Verification items for the finished model (mm, model axes). A direction names the side the tool comes from. Round coordinates to 2 decimals unless told otherwise and drop trailing zeros. Loops run counter-clockwise (first coordinate to the right, second up) from the corner with the lowest first, then second, coordinate; pieces in that order, holes last.
from build123d import *

# Parameters (mm, degrees)
F0_W     = 127
F0_H     = 127
F0_W_2   = 12.7
F0_H_2   = 101.6
F1_DEPTH = 12.7
F2_T     = -2.54


with BuildPart() as f1:
    # F0 (on Top) → F1 (new body)
    with BuildSketch(Plane.XY):
        with Locations((-24.9704163089, 19.614642486)):
            Rectangle(F0_W, F0_H)
        with Locations((-69.4204163089, 19.614642486)):
            Rectangle(F0_W_2, F0_H_2, mode=Mode.SUBTRACT)
        Polygon((-50.3704163089, 6.914642486), (-50.3704163089, 19.614642486), (-50.0745723798, 32.314642486), (-37.0573314681, 32.314642486), (-37.0573314681, 6.914642486), align=None, mode=Mode.SUBTRACT)
        Polygon((-31.3204163089, 32.314642486), (-24.9704163089, 32.314642486), (-18.6204163089, 32.314642486), (-18.6204163089, 6.914642486), (-31.3204163089, 6.914642486), align=None, mode=Mode.SUBTRACT)
        Polygon((0.4295836911, 32.314642486), (0.4295836911, 19.614642486), (0.4295836911, 6.914642486), (-10.8125778138, 6.914642486), (-10.8125778138, 32.314642486), align=None, mode=Mode.SUBTRACT)
        with Locations((19.4795836911, 19.614642486)):
            Rectangle(F0_W_2, F0_H_2, mode=Mode.SUBTRACT)
    extrude(amount=F1_DEPTH)

    # F2
    f2_openings = [f1.faces().sort_by_distance(p)[0] for p in [
        (36.733532, 19.614642, 12.7),
    ]]
    offset(amount=F2_T, openings=f2_openings, kind=Kind.INTERSECTION)


solid = f1.part
1. Scan lines: L1, parallel to X at y = 65.5, z = 10.5; L2, parallel to Y at x = 13.5, z = 5.5; L3, parallel to X at y = 11.5, z = 1.75. Record each from-to range of solid material in increasing order.
2. Section check A-A (y = -2). Enter the section's corners in (x, z).
3. Section check C-C (z = 8.5). Give the number of separate pieces and of enclosed holes in the cut face, then the cut area to 3 significant figures.
4. Release check for a two-part mould opening along X. For faces 4 (the face through (38.53, 19, 6)), 5 (the face through (-12, 21, 0)), 6 (the face through (-60.53, 19, 8)), 7 (the face through (-5, 32.315, 6)) record: released by +X, released by -X, zero draft, split by the parting line, or undercut.
5. Tool access check on faces 1 (the face through (-70, 72.955, 8)), 2 (the face through (-63.07, 19, 6)), 3 (the face through (-13, 20, 12.7)). Record the directions out of +Z, -Z, +X, -X, +Y, -Y that give a thin tool (end or side, any length) a straight path to the whole face; none if there is none.
6. Gauge pin test, flat end, axial feed: P1, Ø4, axis at x = -72, y = 67.5, coming from the +Z side. Record the tip position at first contact, or that the pin passes through.
7. Section check B-B (x = -26.5). Enter the section's corners in (y, z), then the cut area to 3 significant figures.
Taken from the geometry:
1. L1: x = -88.47 to -85.93, -78.31 to -75.77, -63.07 to -60.53, 10.59 to 13.13, 25.83 to 28.37, 35.99 to 38.53
1. L2: y = -43.89 to -41.35, -33.73 to -31.19, 70.41 to 72.95, 80.57 to 83.11
1. L3: x = -88.47 to -75.77, -63.07 to -50.37, -37.06 to -31.32, -18.62 to -10.81, 0.43 to 13.13, 25.83 to 38.53
2. outline: (-88.47, 0) - (-75.77, 0) - (-75.77, 12.7) - (-78.31, 12.7) - (-78.31, 2.54) - (-85.93, 2.54) - (-85.93, 12.7) - (-88.47, 12.7) - close; (-63.07, 0) - (13.13, 0) - (13.13, 12.7) - (10.59, 12.7) - (10.59, 2.54) - (-60.53, 2.54) - (-60.53, 12.7) - (-63.07, 12.7) - close; (25.83, 0) - (38.53, 0) - (38.53, 12.7) - (35.99, 12.7) - (35.99, 2.54) - (28.37, 2.54) - (28.37, 12.7) - (25.83, 12.7) - close
3. separate pieces: 6
3. enclosed holes: 6
3. area: 3,130 mm2
4. face 4: released by +X
4. face 5: zero draft
4. face 6: undercut
4. face 7: undercut
5. face 1: +Z
5. face 2: +Z, -Z
5. face 3: +Z, +X, -X, +Y, -Y
6. P1: passes through
7. outline: (-43.89, 0) - (6.91, 0) - (6.91, 12.7) - (4.37, 12.7) - (4.37, 2.54) - (-41.35, 2.54) - (-41.35, 12.7) - (-43.89, 12.7) - close; (32.31, 0) - (83.11, 0) - (83.11, 12.7) - (80.57, 12.7) - (80.57, 2.54) - (34.85, 2.54) - (34.85, 12.7) - (32.31, 12.7) - close
7. area: 361 mm2
